```python
from build123d import *

# Parameters (mm, degrees)
F0_W     = 210
F0_H     = 297
F0_W_2   = 2.2109179881
F0_H_2   = 19.0238875475
F1_DEPTH = 1


with BuildPart() as f1:
    # F0 (on Top) → F1 (new body)
    with BuildSketch(Plane.XY):
        Rectangle(F0_W, F0_H)
        with BuildLine():
            add(Edge.make_bspline(
                [(-34.1734707151, 16.5652301615), (-31.714813329, 14.1065727754), (-31.714813329, 9.6930641739)],
                knots=[0, 0, 0, 1, 1, 1], degree=2))
            add(Edge.make_bspline(
                [(-31.714813329, 9.6930641739), (-31.714813329, 4.9839337698), (-34.271317368, 2.4919668849)],
                knots=[0, 0, 0, 1, 1, 1], degree=2))
            add(Edge.make_bspline(
                [(-34.271317368, 2.4919668849), (-36.827821407, 0), (-41.628552933, 0)],
                knots=[0, 0, 0, 1, 1, 1], degree=2))
            Line((-41.628552933, 0), (-46.8997811307, 0))
            Line((-46.8997811307, 0), (-46.8997811307, 19.0238875475))
            Line((-46.8997811307, 19.0238875475), (-41.0706188268, 19.0238875475))
            add(Edge.make_bspline(
                [(-41.0706188268, 19.0238875475), (-36.6321281011, 19.0238875475), (-34.1734707151, 16.5652301615)],
                knots=[0, 0, 0, 1, 1, 1], degree=2))
        make_face(mode=Mode.SUBTRACT)
        with Locations((-26.3665569152, 9.5119437738)):
            Rectangle(F0_W_2, F0_H_2, mode=Mode.SUBTRACT)
        with BuildLine():
            Line((-5.1837974715, 19.0238875475), (-5.1837974715, 0))
            Line((-5.1837974715, 0), (-7.7069920117, 0))
            Line((-7.7069920117, 0), (-18.1037193494, 15.963577338))
            Line((-18.1037193494, 15.963577338), (-18.2078115334, 15.963577338))
            add(Edge.make_bspline(
                [(-18.2078115334, 15.963577338), (-17.9996271654, 13.15308837), (-17.9996271654, 10.8130960737)],
                knots=[0, 0, 0, 1, 1, 1], degree=2))
            Line((-17.9996271654, 10.8130960737), (-17.9996271654, 0))
            Line((-17.9996271654, 0), (-20.0439976591, 0))
            Line((-20.0439976591, 0), (-20.0439976591, 19.0238875475))
            Line((-20.0439976591, 19.0238875475), (-17.5457852432, 19.0238875475))
            Line((-17.5457852432, 19.0238875475), (-7.1740400296, 3.1227655199))
            Line((-7.1740400296, 3.1227655199), (-7.0699478456, 3.1227655199))
            add(Edge.make_bspline(
                [(-7.0699478456, 3.1227655199), (-7.0949299698, 3.4725152582), (-7.1865310917, 5.379484069)],
                knots=[0, 0, 0, 1, 1, 1], degree=2))
            add(Edge.make_bspline(
                [(-7.1865310917, 5.379484069), (-7.2781322136, 7.2864528799), (-7.2531500894, 8.1066992898)],
                knots=[0, 0, 0, 1, 1, 1], degree=2))
            Line((-7.2531500894, 8.1066992898), (-7.2531500894, 19.0238875475))
            Line((-7.2531500894, 19.0238875475), (-5.1837974715, 19.0238875475))
        make_face(mode=Mode.SUBTRACT)
        Polygon((21.2181440778, 0), (18.9281160298, 0), (16.558977922, 6.049837734), (8.935266366, 6.049837734), (6.5952740697, 0), (4.3552102701, 0), (11.8748296421, 19.1029976074), (13.735997892, 19.1029976074), align=None, mode=Mode.SUBTRACT)
        Polygon((35.9201241457, 6.3371321618), (35.9201241457, 4.3718717279), (33.0971441156, 4.3718717279), (33.0971441156, 0), (31.0277914978, 0), (31.0277914978, 4.3718717279), (21.776078184, 4.3718717279), (21.776078184, 6.258022102), (30.8071160677, 19.1279797315), (33.0971441156, 19.1279797315), (33.0971441156, 6.3371321618), align=None, mode=Mode.SUBTRACT)
    extrude(amount=F1_DEPTH)


solid = f1.part
```
Geometry check sheet. Reference: the model listing, model coordinates, mm. A direction names the side the tool comes from. Coordinates: 2 decimals unless noted, no trailing zeros. One line per item, written item: value. Start each with the question number.
(1) Scan lines: line 1 along Y through (x, z) = (31.5, 0.2); line 2 along Y through (x, z) = (-37, 0.6). Record each from-to range of solid material in increasing order. Write a range as [from, to].
(2) Tool access check on faces 1 (the face through (26.228, 12.603, 0.493)), 2 (the face through (-1, 2, 1)). Record the directions out of +Z, -Z, +X, -X, +Y, -Y that give a thin tool (end or side, any length) a straight path to the whole face; none if there is none.
(3) Release check for a two-part mould opening along Y. For faces 3 (the face through (-12.43, 11.18, 0.49)), 4 (the face through (-1, 2, 0)) record: released by +Y, released by -Y, zero draft, split by the parting line, or undercut.
Filled sheet:
1. line 1: [-148.5, 0], [19.13, 148.5]
1. line 2: [-148.5, 0.76], [18.36, 148.5]
2. face 1: +Z, -Z
2. face 2: +Z, +X, -X, +Y, -Y
3. face 3: undercut
3. face 4: zero draft
